Verification items for the finished model (mm, model axes). Give positions to 0.01 mm unless a question says otherwise; leave off trailing zeros. Loops run counter-clockwise (first coordinate to the right, second up) from the corner with the lowest first, then second, coordinate; pieces in that order, holes last. Notation, with made-up numbers: (87, -18.75) - (115, -18.75) arc R23 ccw to (115, 4.25) - close; hole circle Ø7 at (39, -5.5). An arc over 180 degrees is marked (long way). One line per item, written item: value. Start each with the question number.
1. Sectioned sample at B-B (x = 0). Record the cut outline in (y, z), plus the area to 3 significant figures.
2. Sectioned sample at A-A (x = -5.75). Record the cut outline in (y, z), plus the area to 3 significant figures.
3. Scan lines: L1, parallel to Y at x = 0, z = 2.3; L2, parallel to X at y = -63.8, z = 3.05; L3, parallel to Y at x = -6, z = 3.65. Record each from-to range of solid material in increasing order. Write a range as [from, to].
4. Sectioned sample at C-C (z = 2.2). Count the separate pieces of the cut face and the enclosed holes in it, plus the area to 3 significant figures.
5. Gauge pin test, flat ends, axial feed: pin 1 (1.1 mm diameter, centred on y = -54, z = 1.5, fed in from -X); pin 2 (1 mm diameter, centred on x = -5.5, z = 2.5, fed in from +Y); pin 3 (1.5 mm diameter, centred on x = -4.5, z = 3.5, fed in from -Y); pin 4 (1.6 mm diameter, centred on x = 0, y = -63.8, fed in from +Z). Record the tip position at first contact, or that the pin passes through.
6. Sectioned sample at D-D (y = -8). Record the cut outline in (x, z), plus the area to 3 significant figures.
from build123d import *

# Parameters (mm, degrees)
SKETCH_1_R          = 2
SKETCH_1_R_2        = 0.6
EXTRUDE_1_DEPTH     = 3.8
SKETCH_2_W          = 4
SKETCH_2_H          = 3.8
EXTRUDE_2_DEPTH     = 10
SKETCH_1_4_R        = 0.6
CUT_EXTRUDE_1_DEPTH = 11.883014288
SKETCH_3_W          = 4
SKETCH_3_H          = 21.9
EXTRUDE_3_DEPTH     = 3.8
SKETCH_5_W          = 7
SKETCH_5_H          = 5
EXTRUDE_4_DEPTH     = 3.8
CUT_EXTRUDE_3_DEPTH = 67.521274792
FILLET_1_R          = 2.5


with BuildPart() as part:
    # 草图1 → 凸台-拉伸1 (new body)
    with BuildSketch(Plane.XY):
        with Locations(Location((0, 0, 0), (0, 0, 180))):
            Circle(SKETCH_1_R)
        Circle(SKETCH_1_R_2, mode=Mode.SUBTRACT)
    extrude(amount=EXTRUDE_1_DEPTH)

    # 草图2 → 凸台-拉伸2 (add)
    with BuildSketch(Plane(origin=(0, 0, 0), x_dir=(1, 0, 0), z_dir=(0, 1, 0))):
        with Locations((0, -1.9)):
            Rectangle(SKETCH_2_W, SKETCH_2_H)
    extrude(amount=-EXTRUDE_2_DEPTH)

    # 草图1<4> → 切除-拉伸1 (cut, through all)
    with BuildSketch(Plane.XY):
        Circle(SKETCH_1_4_R)
    extrude(amount=CUT_EXTRUDE_1_DEPTH, mode=Mode.SUBTRACT)

    # 草图3 → 凸台-拉伸3 (add)
    with BuildSketch(Plane.XY.offset(3.8)):
        with Locations((0, -20.95)):
            Rectangle(SKETCH_3_W, SKETCH_3_H)
    extrude(amount=-EXTRUDE_3_DEPTH)

    # 镜向1: part across plane


with BuildPart() as part_1:
    add(part.part)
    add(part.part.mirror(Plane(origin=(2, -31.9, -22.262299971), x_dir=(0, 0, 1), z_dir=(0, -1, 0))))

    # 草图5 → 凸台-拉伸4 (add)
    with BuildSketch(Plane.XY.offset(3.8)):
        with Locations((-5.5, -31.9)):
            Rectangle(SKETCH_5_W, SKETCH_5_H)
    extrude(amount=-EXTRUDE_4_DEPTH)

    # 草图6 → 切除-拉伸3 (cut, through all)
    with BuildSketch(Plane.XY.offset(3.8)):
        with BuildLine():
            Line((-4, -32.5), (-7, -32.5))
            ThreePointArc((-7, -32.5), (-7.6, -31.9), (-7, -31.3))
            Line((-7, -31.3), (-4, -31.3))
            ThreePointArc((-4, -31.3), (-3.4, -31.9), (-4, -32.5))
        make_face()
    extrude(amount=-CUT_EXTRUDE_3_DEPTH, mode=Mode.SUBTRACT)

    # 圆角1
    fillet_1_edges = [part_1.edges().sort_by_distance(p)[0] for p in [
        (-2, -29.4, 1.9),
        (-2, -34.4, 1.9),
    ]]
    fillet(fillet_1_edges, radius=FILLET_1_R)
    fillet_1_2_edges = [part_1.edges().sort_by_distance(p)[0] for p in [
        (-9, -34.4, 1.9),
        (-9, -29.4, 1.9),
    ]]
    fillet(fillet_1_2_edges, radius=FILLET_1_R - 0.0001)  # a hair under: the kernel refuses the full size


solid = part_1.part
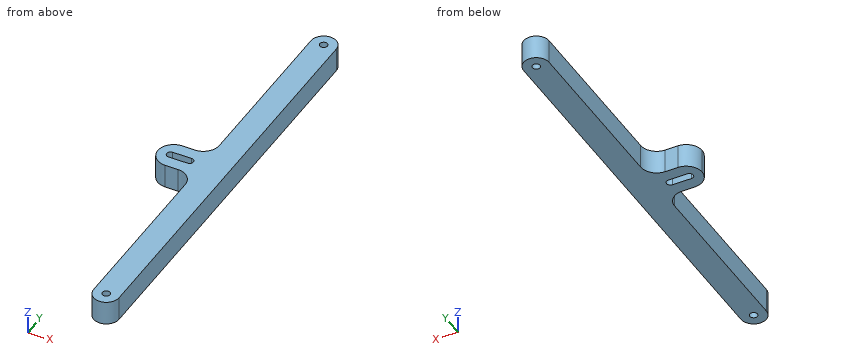
Results are:
1. outline: (-65.8, 0) - (-64.4, 0) - (-64.4, 3.8) - (-65.8, 3.8) - close; (-63.2, 0) - (-0.6, 0) - (-0.6, 3.8) - (-63.2, 3.8) - close; (0.6, 0) - (2, 0) - (2, 3.8) - (0.6, 3.8) - close
1. area: 249 mm^2
2. outline: (-34.4, 0) - (-32.5, 0) - (-32.5, 3.8) - (-34.4, 3.8) - close; (-31.3, 0) - (-29.4, 0) - (-29.4, 3.8) - (-31.3, 3.8) - close
2. area: 14.4 mm^2
3. L1: y = [-65.8, -64.4], [-63.2, -0.6], [0.6, 2]
3. L2: x = [-2, -0.6], [0.6, 2]
3. L3: y = [-34.4, -32.5], [-31.3, -29.4]
4. separate pieces: 1
4. enclosed holes: 3
4. area: 296 mm^2
5. pin 1: stops at x = -2
5. pin 2: stops at y = -29.4
5. pin 3: stops at y = -34.52
5. pin 4: stops at z = 3.8
6. outline: (-2, 0) - (2, 0) - (2, 3.8) - (-2, 3.8) - close
6. area: 15.2 mm^2
